Verification items for the finished model (mm, model axes). A direction names the side the tool comes from. Give positions to 0.01 mm unless a question says otherwise; leave off trailing zeros. Loops run counter-clockwise (first coordinate to the right, second up) from the corner with the lowest first, then second, coordinate; pieces in that order, holes last. Notation, with made-up numbers: M 39.5,38.25 L 66.5,38.25 A35 ccw 66.5,74.25 Z; hole C 25.5,38.5 d10. An arc over 180 degrees is marked long. Use CSV: the item, a comma, the result in double quotes.
from build123d import *

# Parameters (mm, degrees)
BOSS_EXTRUDE1_DEPTH      = 101.6
BOSS_EXTRUDE1_DEPTH_BACK = 101.6
SKETCH1_R                = 57.15
SKETCH1_R_2              = 50.8
CUT_EXTRUDE3_DEPTH       = 130.826056707
CUT_EXTRUDE3_DEPTH_BACK  = 130.826056707
SKETCH3_W                = 40
SKETCH3_H                = 10
SKETCH5_W                = 40
SKETCH5_H                = 35
CUT_EXTRUDE5_DEPTH       = 18.15
CUT_EXTRUDE6_DEPTH       = 130.826056707
CUT_EXTRUDE6_DEPTH_BACK  = 130.826056707
SKETCH6_W                = 252.16572489
SKETCH6_H                = 244.887597008
SKETCH6_R                = 101.6


with BuildPart() as part:
    # Sketch1 → Boss-Extrude1 (new, two sides: drawn at the far end of the back side and taken through both)
    with BuildSketch(Plane(origin=(0, 0, 0), x_dir=(0, 0, -1), z_dir=(1, 0, 0)).offset(-BOSS_EXTRUDE1_DEPTH_BACK)):
        Circle(SKETCH1_R)
        Circle(SKETCH1_R_2, mode=Mode.SUBTRACT)
    extrude(amount=BOSS_EXTRUDE1_DEPTH + BOSS_EXTRUDE1_DEPTH_BACK)

    # Sketch3 → Cut-Extrude3 (cut, two sides: drawn at the far end of the back side and taken through both)
    with BuildSketch(Plane.XY.offset(-CUT_EXTRUDE3_DEPTH_BACK)):
        with Locations((20, 54)):
            Rectangle(SKETCH3_W, SKETCH3_H)
    extrude(amount=CUT_EXTRUDE3_DEPTH + CUT_EXTRUDE3_DEPTH_BACK, mode=Mode.SUBTRACT)

    # Sketch5 → Cut-Extrude5 (cut)
    with BuildSketch(Plane(origin=(0, 49, 0), x_dir=(1, 0, 0), z_dir=(0, 1, 0))):
        with Locations((20, 0)):
            Rectangle(SKETCH5_W, SKETCH5_H)
    extrude(amount=-CUT_EXTRUDE5_DEPTH, mode=Mode.SUBTRACT)

    # Sketch6 → Cut-Extrude6 (cut, two sides: drawn at the far end of the back side and taken through both)
    with BuildSketch(Plane(origin=(0, 0, 0), x_dir=(1, 0, 0), z_dir=(0, 1, 0)).offset(-CUT_EXTRUDE6_DEPTH_BACK)):
        Rectangle(SKETCH6_W, SKETCH6_H)
        Circle(SKETCH6_R, mode=Mode.SUBTRACT)
    extrude(amount=CUT_EXTRUDE6_DEPTH + CUT_EXTRUDE6_DEPTH_BACK, mode=Mode.SUBTRACT)


solid = part.part
(1) Tool access check on faces 1 (the flat face through (20, 49, -24)), 2 (the cylindrical face through (-1.422, -34.775, 45.352)). Record the directions out of +Z, -Z, +X, -X, +Y, -Y that give a thin tool (end or side, any length) a straight path to the whole face; none if there is none.
Calculated:
face 1,"+Z, -Z, +Y"
face 2,"+X, -X"
(2) Section check D-D on x = -81.5. Record the cut outline in (y, z), plus the area to 3 significant figures.
Calculated:
outline,"C 0,0 d114.3; hole C 0,0 d101.6"
area,"2,150 mm²"
(3) Scan lines: L1, parallel to Y at x = -17, z = 0; L2, parallel to Y at x = 29, z = 0. Record each from-to range of solid material in increasing order. Write a range as from..to.
Calculated:
L1,"y = -57.15..-50.8, 50.8..57.15"
L2,"y = -57.15..-50.8"
(4) Section check C-C on z = 27. Record the cut outline in (x, y).
Calculated:
outline,"M -97.95,-50.37 L 97.95,-50.37 L 97.95,-43.03 L -97.95,-43.03 Z; M -97.95,43.03 L 97.95,43.03 L 97.95,50.37 L 40,50.37 L 40,49 L 0,49 L 0,50.37 L -97.95,50.37 Z"
(5) Section check A-A on z = 0. Record the cut outline in (x, y).
Calculated:
outline,"M -101.6,-57.15 L 101.6,-57.15 L 101.6,-50.8 L -101.6,-50.8 Z; M -101.6,50.8 L 0,50.8 L 0,57.15 L -101.6,57.15 Z; M 40,50.8 L 101.6,50.8 L 101.6,57.15 L 40,57.15 Z"
(6) Mould release check, pull along X, two halves, no side actions. Record for faces 3 (the flat face through (20, 49, 23)), 4 (the cylindrical face through (101.6, -51.1, 0.3)), 5 (the cylindrical face through (-101.6, -51.1, -0.3)): released by +X, released by -X, zero draft, split by the parting line, or undercut.
Calculated:
face 3,"undercut"
face 4,"released by +X"
face 5,"released by -X"
(7) Depth check by flat-ended pin: pin 1 Ø1.5 at (x, z) = (28.5, 30.5) entering from +Y; pin 2 Ø9.5 at (x, z) = (16.5, -22) entering from +Y; pin 3 Ø4 at (x, y) = (12, 32.5) entering from +Z. Enter the tip coordinate at first touch or a pass-through.
Calculated:
pin 1,"stops at y = 48.8"
pin 2,"stops at y = 49"
pin 3,"stops at z = 48.33"
(8) Section check B-B on y = 28. Record the cut outline in (x, z).
Calculated:
outline,"M -92.34,-42.39 A101.6 ccw -88.55,-49.82 L 88.55,-49.82 A101.6 ccw 92.34,-42.39 Z; M -92.34,42.39 L 92.34,42.39 A101.6 ccw 88.55,49.82 L -88.55,49.82 A101.6 ccw Z"
